Job drawing, mm, ordinate dimensions from the low corner. One solid piece. Give positions to 0.01 mm unless a question says otherwise; leave off trailing zeros. Write each loop counter-clockwise with the first axis right and the second up, starting at its lowest first coordinate (ties: lowest second). Pieces come first, ordered by that corner, then holes. Notation, with made-up numbers: (-10, 37.25) -> (34, 37.25) arc R26 ccw to (34, 51.25) -> close; hole circle Ø5 at (62, -19.75). An arc over 180 degrees is marked (long way). Put each result on its own line as item: value. Start each with the question number.
Item 1: Slice it at A-A, the plane y = 12.7. List the corners of the cut face in (x, z) (1 decimal), plus the area to 3 significant figures.
Item 2: Drill centre line: line 1 along Y through (x, z) = (63.5, 7.25). Where is it in solid material? Low to high.
Item 3: Flat gauge pin, fed straight in: pin 1 Ø4 at (y, z) = (17, 3.5) entering from -X. Where does the tip first touch, or does it go through?
Item 4: Slice it at B-B, the plane x = 38.1. List the corners of the cut face in (y, z) (1 decimal).
Item 5: Slice it at C-C, the plane z = 7.75. List the corners of the cut face in (x, y), plus the area to 3 significant figures.
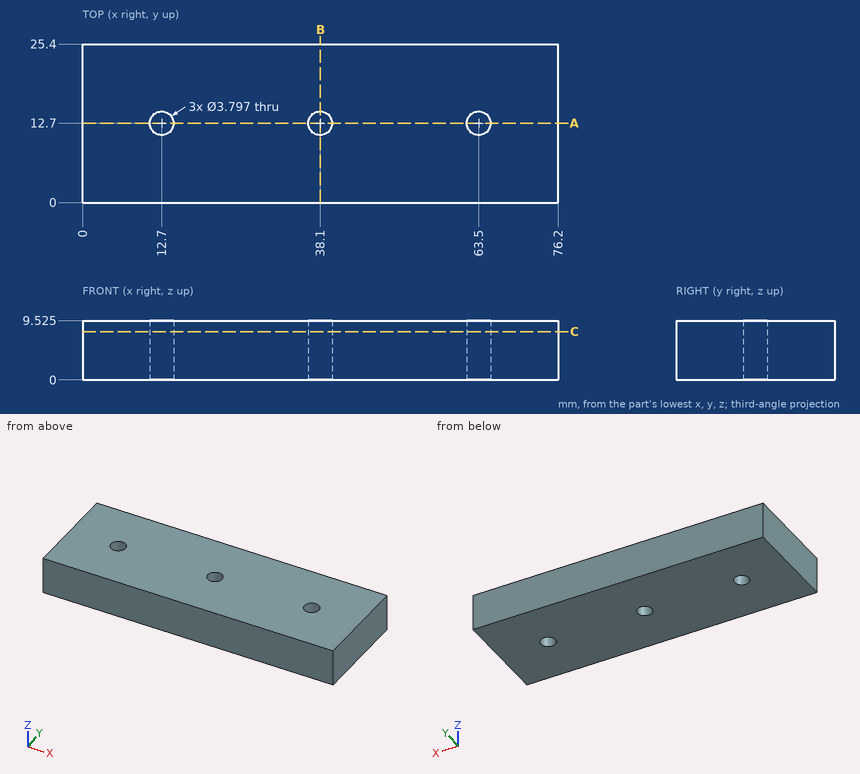
Values follow:
1. outline: (0, 0) -> (10.8, 0) -> (10.8, 9.5) -> (0, 9.5) -> close; (14.6, 0) -> (36.2, 0) -> (36.2, 9.5) -> (14.6, 9.5) -> close; (40, 0) -> (61.6, 0) -> (61.6, 9.5) -> (40, 9.5) -> close; (65.4, 0) -> (76.2, 0) -> (76.2, 9.5) -> (65.4, 9.5) -> close
1. area: 617 mm2
2. line 1: 0 to 10.8, 14.6 to 25.4
3. pin 1: x = 0
4. outline: (0, 0) -> (10.8, 0) -> (10.8, 9.5) -> (0, 9.5) -> close; (14.6, 0) -> (25.4, 0) -> (25.4, 9.5) -> (14.6, 9.5) -> close
5. outline: (0, 0) -> (76.2, 0) -> (76.2, 25.4) -> (0, 25.4) -> close; hole circle Ø3.8 at (12.7, 12.7); hole circle Ø3.8 at (38.1, 12.7); hole circle Ø3.8 at (63.5, 12.7)
5. area: 1,900 mm2
